Input: part model. Units: mm. Frame: model coordinates. A direction names the side the tool comes from. Coordinates: 2 decimals unless noted, no trailing zeros. Order: outer loops, then holes, each group sorted by start corner. A loop starts at its lowest first (then second) coordinate and runs counter-clockwise, first axis right, second up. Notation, with made-up numbers: M 3.5,-13.5 L 21.5,-13.5 A21 ccw 21.5,9.5 Z; hole C 66,18.5 d1. An arc over 180 degrees is marked long. One line per item, written item: value.
```python
from build123d import *

# Parameters (mm, degrees)
BOSS_EXTRUDE1_DEPTH = 6
SKETCH3_R           = 1.5
CUT_EXTRUDE2_DEPTH  = 47.916521486
SKETCH4_R           = 1.5
CUT_EXTRUDE3_DEPTH  = 11


with BuildPart() as part:
    # Sketch1 → Boss-Extrude1 (new body)
    with BuildSketch(Plane(origin=(0, 0, 0), x_dir=(1, 0, 0), z_dir=(0, 1, 0))):
        with BuildLine():
            Line((2, 43.916521486), (2, 23.916521486))
            ThreePointArc((2, 23.916521486), (24, 0), (2, -23.916521486))
            Line((2, -23.916521486), (2, -43.916521486))
            Line((2, -43.916521486), (12, -43.916521486))
            Line((12, -43.916521486), (12, -31.811947441))
            ThreePointArc((12, -31.811947441), (27.082954224, -20.55513538), (33.867388444, -3))
            Line((33.867388444, -3), (45.867388444, -3))
            Line((45.867388444, -3), (45.867388444, 3))
            Line((45.867388444, 3), (33.867388444, 3))
            ThreePointArc((33.867388444, 3), (27.082954224, 20.55513538), (12, 31.811947441))
            Line((12, 31.811947441), (12, 43.916521486))
            Line((12, 43.916521486), (2, 43.916521486))
        make_face()
    extrude(amount=BOSS_EXTRUDE1_DEPTH)

    # Sketch3 → Cut-Extrude2 (cut, through all)
    with BuildSketch(Plane(origin=(0, 0, -3), x_dir=(-1, 0, 0), z_dir=(0, 0, -1))):
        with Locations((-41.367388444, 3)):
            Circle(SKETCH3_R)
    extrude(amount=-CUT_EXTRUDE2_DEPTH, mode=Mode.SUBTRACT)

    # Sketch4 → Cut-Extrude3 (cut, through all)
    with BuildSketch(Plane(origin=(12, 0, 0), x_dir=(0, 0, -1), z_dir=(1, 0, 0))):
        with Locations((-38.916521486, 3)):
            Circle(SKETCH4_R)
    cut_extrude3 = extrude(amount=-CUT_EXTRUDE3_DEPTH, mode=Mode.SUBTRACT)

    # Mirror1: Cut-Extrude3 across plane
    add(cut_extrude3.mirror(Plane.XY), mode=Mode.SUBTRACT)


solid = part.part
```
(1) First-contact query: pin 1 (1.8 mm diameter, centred on y = 4.5, z = -39, fed in from +X); pin 2 (2 mm diameter, centred on y = 5.5, z = -17.5, fed in from +X); pin 3 (3 mm diameter, centred on x = 37.5, y = 3, fed in from -Z). Flat tips, straight axial feed; report the tip coordinate or a pass-through.
Data:
pin 1: stops at x = 12
pin 2: stops at x = 29.73
pin 3: stops at z = -3
(2) Cut plane B-B on y = 3. Output: boundary loops of the cut face in (x, z).
Data:
outline: M 2,-43.92 L 12,-43.92 L 12,-40.42 L 2,-40.42 Z; M 2,-37.42 L 12,-37.42 L 12,-31.81 A34 ccw 33.87,-3 L 39.87,-3 L 39.87,3 L 33.87,3 A34 ccw 12,31.81 L 12,37.42 L 2,37.42 L 2,23.92 A24 cw 2,-23.92 Z; M 2,40.42 L 12,40.42 L 12,43.92 L 2,43.92 Z; M 42.87,-3 L 45.87,-3 L 45.87,3 L 42.87,3 Z
(3) Cut plane D-D on z = -17.5. Output: boundary loops of the cut face in (x, y), plus the area to 3 significant figures.
Data:
outline: M 16.42,0 L 29.15,0 L 29.15,6 L 16.42,6 Z
area: 76.4 mm2
(4) Ray query, line 1 (X direction, y = 5.1, z = -38); line 2 (Z direction, x = 37, y = 4.3); line 3 (Z direction, x = 18, y = 1.6). Return the intervals inside material, ascending. Write a range as from..to.
Data:
line 1: x = 2..12
line 2: z = -3..3
line 3: z = -28.84..-15.87, 15.87..28.84
(5) Cut plane A-A on x = 8. Output: boundary loops of the cut face in (y, z).
Data:
outline: M 0,-43.92 L 6,-43.92 L 6,-22.63 L 0,-22.63 Z; M 0,22.63 L 6,22.63 L 6,43.92 L 0,43.92 Z; hole C 3,-38.92 d3; hole C 3,38.92 d3
(6) Draft query along Z for faces 1 (the cylindrical face through (7.07, 2.09, -40.11)), 2 (the flat face through (12, 3, -36)), 3 (the flat face through (40, 2, 3)). Return one class per face: released by +Z, released by -Z, zero draft, split by the parting line, or undercut.
Data:
face 1: undercut
face 2: zero draft
face 3: released by +Z
(7) Access query for faces 4 (the flat face through (12, 3, 37)), 5 (the flat face through (40, 2, -3)), 6 (the flat face through (24, 0, -3)). Directions: +Z, -Z, +X, -X, +Y, -Y. A direction counts if a zero-diameter tool reaches every point of the face in a straight line with its end or side. Return the directions, or none.
Data:
face 4: +Z, +X, +Y, -Y
face 5: -Z, +X, +Y, -Y
face 6: +Z, -Z, +X, -X, -Y
(8) Cut plane C-C on x = 38.5. Output: boundary loops of the cut face in (y, z).
Data:
outline: M 0,-3 L 6,-3 L 6,3 L 0,3 Z
